from build123d import *

# Parameters (mm, degrees)
F0_R     = 11
F1_DEPTH = 3
F2_R     = 5.5
F3_DEPTH = 0.45
F4_R     = 4.05
F5_DEPTH = 3
F6_SIZE  = 0.25
F8_SIZE  = 0.5


# Not quite as in the source:
# - a fillet or chamfer that OpenCascade refuses, or shapes differently, is made with other operations: its cross-section is extruded or revolved along the edge and cut away or added


with BuildPart() as f1:
    # F0 (on Top) → F1 (new body)
    with BuildSketch(Plane.XY):
        Circle(F0_R)
    extrude(amount=F1_DEPTH)

    # F2 (on face) → F3 (join)
    with BuildSketch(Plane.XY.offset(3)):
        Circle(F2_R)
    extrude(amount=F3_DEPTH)

    # F4 (on face) → F5 (join)
    with BuildSketch(Plane.XY.offset(3.45)):
        Circle(F4_R)
    extrude(amount=F5_DEPTH)

    # F6
    f6_edges = [f1.edges().sort_by_distance(p)[0] for p in [
        (-4.05, 0, 6.45),
    ]]
    chamfer(f6_edges, length=F6_SIZE)

    # F7: chamfer of 0.5 on 1 edges, made by hand


with BuildPart() as f7_tool2:
    # F7_s3 → F7_t4 (revolve)
    with BuildSketch(Plane.XZ):
        Polygon((5, 3.45), (5.5, 2.95), (5.5, 3.45), align=None)
    revolve(axis=Axis((0, 0, 3.45), (0, 0, 1)))

    split(bisect_by=Plane.XY.offset(3), keep=Keep.TOP)


with BuildPart() as f1_1:
    add(f1.part)

    # F7_t1: cut F7_tool2
    add(f7_tool2.part, mode=Mode.SUBTRACT)

    # F8
    f8_edges = [f1_1.edges().sort_by_distance(p)[0] for p in [
        (-11, 0, 0),
        (-11, 0, 3),
    ]]
    chamfer(f8_edges, length=F8_SIZE)


solid = f1_1.part
Input: part model. Units: mm. Frame: model coordinates. A direction names the side the tool comes from. Coordinates: 2 decimals unless noted, no trailing zeros. Loops run counter-clockwise (first coordinate to the right, second up) from the corner with the lowest first, then second, coordinate; pieces in that order, holes last.
Q1. Cut plane A-A (x = 0). Output: boundary loops of the cut face in (y, z).
Q2. Contact query for flat-ended pins moving along their axis: pin 1 (1 mm diameter, centred on y = -8, z = 2.5, fed in from +X); pin 2 (1 mm diameter, centred on x = 5.5, z = 4.5, fed in from -Y); pin 3 (2 mm diameter, centred on x = -8, y = -3.5, fed in from +Z); pin 4 (3 mm diameter, centred on x = -6.5, z = 3, fed in from +Y). Output: stop coordinate, or through.
Q3. Set-up query: faces 1 (the face through (5, -5, 3)), 2 (the face through (0, 0, 6.45)). Return all of +Z, -Z, +X, -X, +Y, -Y with unobstructed straight access to the full face (end or side cutting, diameter ignored); none if empty.
Q4. Cut plane D-D (z = 5). Output: boundary loops of the cut face in (x, y), then the cut area to 3 significant figures.
Q5. Cut plane C-C (z = 1). Output: boundary loops of the cut face in (x, y).
Q6. Material intervals for line 1 (Z direction, x = 7.5, y = -7.25); line 2 (Z direction, x = 9.75, y = -4.75); line 3 (X direction, y = 3.75, z = 1), sorted ascending.
Working result:
1. outline: (-11, 0.5) - (-10.5, 0) - (10.5, 0) - (11, 0.5) - (11, 2.5) - (10.5, 3) - (5.45, 3) - (5, 3.45) - (4.05, 3.45) - (4.05, 6.2) - (3.8, 6.45) - (-3.8, 6.45) - (-4.05, 6.2) - (-4.05, 3.45) - (-5, 3.45) - (-5.45, 3) - (-10.5, 3) - (-11, 2.5) - close
2. pin 1: stops at x = 8.05
2. pin 2: passes through
2. pin 3: stops at z = 3
2. pin 4: stops at y = 9.75
3. face 1: +Z
3. face 2: +Z, +X, -X, +Y, -Y
4. outline: circle Ø8.1 at (0, 0)
4. area: 51.5 mm2
5. outline: circle Ø22 at (0, 0)
6. line 1: z = 0 to 3
6. line 2: z = 0.35 to 2.65
6. line 3: x = -10.34 to 10.34
